Model file for the job. Use its own axes, mm. Face numbers are marked on the shaded views. Coordinates: 2 decimals unless noted, no trailing zeros. Write each loop counter-clockwise with the first axis right and the second up, starting at its lowest first coordinate (ties: lowest second). Pieces come first, ordered by that corner, then holes.
Q1. Drill centre lines: probe 1 along Y at (x, z) = (3.5, 2.75); probe 2 along Y at (x, z) = (-3, -2); probe 3 along X at (y, z) = (2.15, 0). Where is each one in solid material? Low to high.
Q2. Pin check, flat tips, straight feed: P1, Ø5, axis at x = -3.5, y = 21, coming from the +Z side; P2, Ø2.5, axis at x = 0, z = 0, coming from the +Y side; P3, Ø2, axis at y = 52, z = -3, coming from the -X side. Stop position of each tip, or through.
Q3. Band-saw the part on A-A, the plane y = 23. Write the cut outline in (x, z), plus the area to 3 significant figures.
Q4. Pull direction X, two halves, no side cores. Call the marked faces 1 and 2: released by +X, released by -X, zero draft, split by the parting line, or undercut.
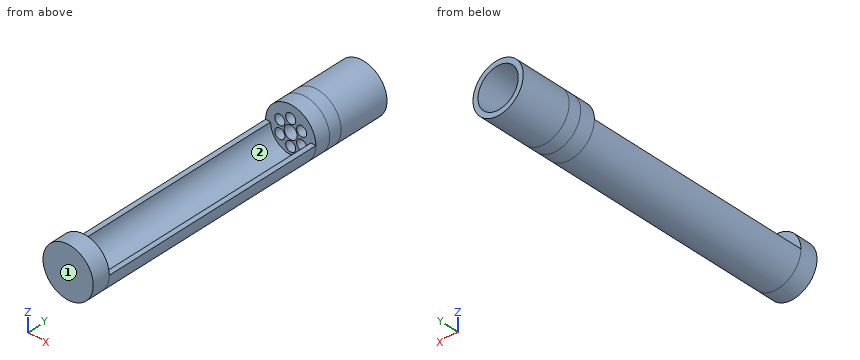
from build123d import *

# Parameters (mm, degrees)
SKETCH1_R           = 5
BOSS_EXTRUDE1_DEPTH = 3.5
SKETCH2_R           = 2.6
CUT_EXTRUDE1_DEPTH  = 2.5
BOSS_EXTRUDE2_DEPTH = 45
SKETCH4_R           = 5
SKETCH4_R_2         = 1.3
BOSS_EXTRUDE3_DEPTH = 3
SKETCH7_R           = 1
CUT_EXTRUDE2_DEPTH  = 2
CIRPATTERN1_COUNT   = 6
SKETCH8_R           = 5
SKETCH8_R_2         = 2.6
BOSS_EXTRUDE4_DEPTH = 2.5
SKETCH9_R           = 0.2
CUT_EXTRUDE3_DEPTH  = 50.012753442
CIRPATTERN2_COUNT   = 6
SKETCH10_R          = 5
SKETCH10_R_2        = 4
BOSS_EXTRUDE5_DEPTH = 10


with BuildPart() as part:
    # Sketch1 → Boss-Extrude1 (new body)
    with BuildSketch(Plane(origin=(0, 0, 0), x_dir=(1, 0, 0), z_dir=(0, 1, 0))):
        with Locations(Location((0, 0, 0), (0, 0, 270))):
            Circle(SKETCH1_R)
    extrude(amount=BOSS_EXTRUDE1_DEPTH)

    # Sketch2 → Cut-Extrude1 (cut)
    with BuildSketch(Plane(origin=(0, 3.5, 0), x_dir=(1, 0, 0), z_dir=(0, 1, 0))):
        with Locations(Location((0, 0, 0), (0, 0, 270))):
            Circle(SKETCH2_R)
    extrude(amount=-CUT_EXTRUDE1_DEPTH, mode=Mode.SUBTRACT)

    # Sketch3 → Boss-Extrude2 (add)
    with BuildSketch(Plane(origin=(0, 3.5, 0), x_dir=(1, 0, 0), z_dir=(0, 1, 0))):
        with BuildLine():
            Line((5, 0), (4, 0))
            ThreePointArc((4, 0), (0, 4), (-4, 0))
            Line((-4, 0), (-5, 0))
            ThreePointArc((-5, 0), (0, 5), (5, 0))
        make_face()
    extrude(amount=BOSS_EXTRUDE2_DEPTH)

    # Sketch4 → Boss-Extrude3 (add)
    with BuildSketch(Plane(origin=(0, 48.5, 0), x_dir=(1, 0, 0), z_dir=(0, 1, 0))):
        with Locations(Location((0, 0, 0), (0, 0, 270))):
            Circle(SKETCH4_R)
        with Locations(Location((0, 0, 0), (0, 0, 270))):
            Circle(SKETCH4_R_2, mode=Mode.SUBTRACT)
    extrude(amount=BOSS_EXTRUDE3_DEPTH)

    # Sketch7 → Cut-Extrude2 (cut)
    with BuildSketch(Plane.XZ.offset(-48.5)):
        with Locations(Location((0, 2.5, 0), (0, 0, 270))):
            Circle(SKETCH7_R)
    cut_extrude2 = extrude(amount=-CUT_EXTRUDE2_DEPTH, mode=Mode.SUBTRACT)

    # CirPattern1: Cut-Extrude2 ×6 about axis
    cirpattern1_axis = Axis((0, 0, 0), (0, 1, 0))
    for i in range(1, CIRPATTERN1_COUNT):
        add(cut_extrude2.rotate(cirpattern1_axis, i * 360 / CIRPATTERN1_COUNT), mode=Mode.SUBTRACT)

    # Sketch8 → Boss-Extrude4 (add)
    with BuildSketch(Plane(origin=(0, 51.5, 0), x_dir=(1, 0, 0), z_dir=(0, 1, 0))):
        with Locations(Location((0, 0, 0), (0, 0, 270))):
            Circle(SKETCH8_R)
        with Locations(Location((0, 0, 0), (0, 0, 270))):
            Circle(SKETCH8_R_2, mode=Mode.SUBTRACT)
    extrude(amount=BOSS_EXTRUDE4_DEPTH)

    # Sketch9 → Cut-Extrude3 (cut, through all)
    with BuildSketch(Plane.XZ.offset(-48.5)):
        with Locations(Location((0, 3, 0), (0, 0, 270))):
            Circle(SKETCH9_R)
    cut_extrude3 = extrude(amount=-CUT_EXTRUDE3_DEPTH, mode=Mode.SUBTRACT)

    # CirPattern2: Cut-Extrude3 ×6 about axis
    cirpattern2_axis = Axis((0, 0, 0), (0, 1, 0))
    for i in range(1, CIRPATTERN2_COUNT):
        add(cut_extrude3.rotate(cirpattern2_axis, i * 360 / CIRPATTERN2_COUNT), mode=Mode.SUBTRACT)

    # Sketch10 → Boss-Extrude5 (add)
    with BuildSketch(Plane(origin=(0, 54, 0), x_dir=(1, 0, 0), z_dir=(0, 1, 0))):
        with Locations(Location((0, 0, 0), (0, 0, 270))):
            Circle(SKETCH10_R)
        with Locations(Location((0, 0, 0), (0, 0, 270))):
            Circle(SKETCH10_R_2, mode=Mode.SUBTRACT)
    extrude(amount=BOSS_EXTRUDE5_DEPTH)


solid = part.part
Answer sheet:
1. probe 1: y = 0 to 3.5, 48.5 to 64
1. probe 2: y = 0 to 3.5, 48.5 to 54
1. probe 3: x = -5 to -2.6, 2.6 to 5
2. P1: stops at z = 0
2. P2: stops at y = 1
2. P3: stops at x = -4.58
3. outline: (-5, 0) arc R5 ccw to (5, 0) - (4, 0) arc R4 cw to (-4, 0) - close
3. area: 14.1 mm2
4. face 1: zero draft
4. face 2: undercut
